```python
from build123d import *

# Parameters (mm, degrees)
SKETCH1_W           = 50
SKETCH1_H           = 20.3
BOSS_EXTRUDE1_DEPTH = 15
SKETCH2_W           = 50
SKETCH2_H           = 35
BOSS_EXTRUDE2_DEPTH = 15
SKETCH3_W           = 1.3
SKETCH3_H           = 50.3
CUT_EXTRUDE1_DEPTH  = 22
BOSS_EXTRUDE3_DEPTH = 25


with BuildPart() as part:
    # Sketch1 → Boss-Extrude1 (new body)
    with BuildSketch(Plane(origin=(0, 0, 0), x_dir=(1, 0, 0), z_dir=(0, 1, 0))):
        with Locations((25, 10.15)):
            Rectangle(SKETCH1_W, SKETCH1_H)
    extrude(amount=BOSS_EXTRUDE1_DEPTH)

    # Sketch2 → Boss-Extrude2 (add)
    with BuildSketch(Plane.XY):
        with Locations((25, 17.5)):
            Rectangle(SKETCH2_W, SKETCH2_H)
    boss_extrude2 = extrude(amount=BOSS_EXTRUDE2_DEPTH)

    # Mirror1: Boss-Extrude2 across plane
    add(boss_extrude2.mirror(Plane(origin=(0, 0, -10.15), x_dir=(1, 0, 0), z_dir=(0, 0, -1))))

    # Sketch3 → Cut-Extrude1 (cut)
    with BuildSketch(Plane(origin=(0, 35, 0), x_dir=(1, 0, 0), z_dir=(0, 1, 0))):
        with Locations((25, 10.15)):
            Rectangle(SKETCH3_W, SKETCH3_H)
    extrude(amount=-CUT_EXTRUDE1_DEPTH, mode=Mode.SUBTRACT)

    # Sketch4 → Boss-Extrude3 (add)
    with BuildSketch(Plane.ZY):
        Polygon((-35.3, 0), (15, 0), (15, 35), (0, 35), (0, 15), (-20.3, 15), (-20.3, 35), (-35.3, 35), align=None)
    extrude(amount=BOSS_EXTRUDE3_DEPTH)


solid = part.part
```
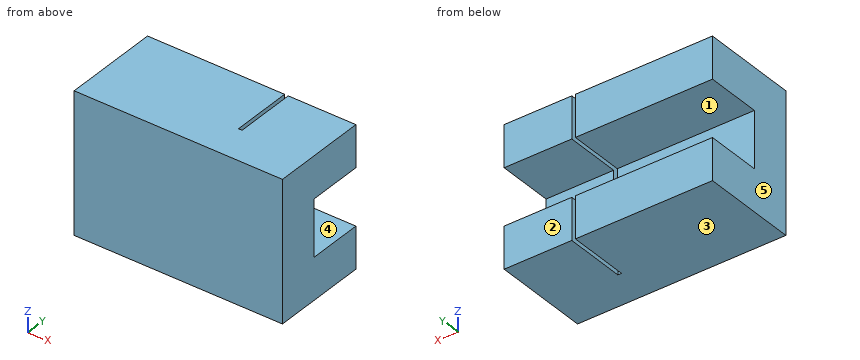
Could you check a few things on this model? Use its own coordinates, in mm. Face numbers are marked on the shaded views. A direction names the side the tool comes from. Give positions to 0.01 mm unless a question says otherwise; leave off trailing zeros. Loops run counter-clockwise (first coordinate to the right, second up) from the corner with the lowest first, then second, coordinate; pieces in that order, holes last. Notation, with made-up numbers: (41, -12) - (78, -12) arc R23 cw to (78, 7) - close; hole circle Ø5 at (-32.75, 79.5). An arc over 180 degrees is marked (long way). Use one line per item in the form item = value.
1. I'm going to push a flat-ended pin straight in: pin 1 Ø4 at (y, z) = (19.5, -17) entering from -X. Where does the tip first touch, or does it pass through?
Response values:
pin_1 = through
2. I want a section at C-C (x = 38). Please give me the cut outline in (y, z).
Response values:
outline = (0, -35.3) - (35, -35.3) - (35, -20.3) - (15, -20.3) - (15, 0) - (35, 0) - (35, 15) - (0, 15) - close
3. On a 3-axis mill with a long thin cutter (end or side, diameter ignored), from which of +Z, -Z, +X, -X, +Y, -Y can I reach the whole of each face in a straight line? I mean the marked faces 4 and 5. Say none if no direction works.
Response values:
face_4 = +X, -X, +Y
face_5 = +Z, -Z, -X, +Y, -Y
4. I want a section at A-A (y = 25). Please give me the cut outline in (x, z), and give its area (3 significant figures).
Response values:
outline = (-25, -35.3) - (24.35, -35.3) - (24.35, -20.3) - (-25, -20.3) - close; (-25, 0) - (24.35, 0) - (24.35, 15) - (-25, 15) - close; (25.65, -35.3) - (50, -35.3) - (50, -20.3) - (25.65, -20.3) - close; (25.65, 0) - (50, 0) - (50, 15) - (25.65, 15) - close
area = 2,210 mm²
5. I want a section at B-B (z = -14.5). Please give me the cut outline in (x, y).
Response values:
outline = (-25, 0) - (50, 0) - (50, 15) - (25.65, 15) - (25.65, 13) - (24.35, 13) - (24.35, 15) - (-25, 15) - close
6. Thinking about a two-plate mould opening in Z: for the marked faces 1, 2 and 3, which applies, released by +Z, released by -Z, zero draft, split by the parting line, or undercut?
Response values:
face_1 = undercut
face_2 = zero draft
face_3 = released by -Z
7. I need wall thicknesses on probe 1 along X at (y, z) = (26, 7.5); probe 2 along Z at (x, y) = (-15.5, 16.5); probe 3 along Y at (x, z) = (22.5, -4). Which ranges of each line are inside material? Lowest first, please.
Response values:
probe_1 = -25 to 24.35, 25.65 to 50
probe_2 = -35.3 to -20.3, 0 to 15
probe_3 = 0 to 15
